from build123d import *

# Parameters (mm, degrees)
SKETCH1_W           = 85
SKETCH1_H           = 20
BOSS_EXTRUDE1_DEPTH = 3
SKETCH2_W           = 3
SKETCH2_H           = 20
BOSS_EXTRUDE2_DEPTH = 12
SKETCH3_W           = 49.5
SKETCH3_H           = 20
BOSS_EXTRUDE3_DEPTH = 3
SKETCH4_W           = 43.5
SKETCH4_H           = 3
CUT_EXTRUDE1_DEPTH  = 50.307707308
SKETCH5_R           = 3.1
CUT_EXTRUDE2_DEPTH  = 48.22552276
SKETCH6_R           = 1.6
CUT_EXTRUDE3_DEPTH  = 48.22552276
FILLET1_R           = 3


with BuildPart() as part:
    # Sketch1 → Boss-Extrude1 (new body)
    with BuildSketch(Plane.XY):
        Rectangle(SKETCH1_W, SKETCH1_H)
    extrude(amount=BOSS_EXTRUDE1_DEPTH)

    # Sketch2 → Boss-Extrude2 (add)
    with BuildSketch(Plane(origin=(0, 0, 0), x_dir=(-1, 0, 0), z_dir=(0, 0, -1))):
        with Locations((-23.25, 0)):
            Rectangle(SKETCH2_W, SKETCH2_H)
        with Locations((23.25, 0)):
            Rectangle(SKETCH2_W, SKETCH2_H)
    extrude(amount=BOSS_EXTRUDE2_DEPTH)

    # Sketch3 → Boss-Extrude3 (add)
    with BuildSketch(Plane(origin=(0, 0, -12), x_dir=(-1, 0, 0), z_dir=(0, 0, -1))):
        Rectangle(SKETCH3_W, SKETCH3_H)
    extrude(amount=BOSS_EXTRUDE3_DEPTH)

    # Sketch4 → Cut-Extrude1 (cut, through all)
    with BuildSketch(Plane.XZ.offset(10)):
        with Locations((0, 1.5)):
            Rectangle(SKETCH4_W, SKETCH4_H)
    extrude(amount=-CUT_EXTRUDE1_DEPTH, mode=Mode.SUBTRACT)

    # Sketch5 → Cut-Extrude2 (cut, through all)
    with BuildSketch(Plane(origin=(0, 0, -15), x_dir=(-1, 0, 0), z_dir=(0, 0, -1))):
        Circle(SKETCH5_R)
    extrude(amount=-CUT_EXTRUDE2_DEPTH, mode=Mode.SUBTRACT)

    # Sketch6 → Cut-Extrude3 (cut, through all)
    with BuildSketch(Plane.XY.offset(3)):
        with Locations((32.380648159, 0.030992543)):
            Circle(SKETCH6_R)
        with Locations((-32.619351841, 0.030992543)):
            Circle(SKETCH6_R)
    extrude(amount=-CUT_EXTRUDE3_DEPTH, mode=Mode.SUBTRACT)

    # Fillet1
    fillet1_edges = [part.edges().sort_by_distance(p)[0] for p in [
        (24.75, 0, -15),
        (-24.75, 0, -15),
        (42.5, -10, 1.5),
        (-42.5, -10, 1.5),
        (-42.5, 10, 1.5),
        (42.5, 10, 1.5),
    ]]
    fillet(fillet1_edges, radius=FILLET1_R)


solid = part.part
Model file for the job. Use its own axes, mm. A direction names the side the tool comes from. Give positions to 0.01 mm unless a question says otherwise; leave off trailing zeros. Loops run counter-clockwise (first coordinate to the right, second up) from the corner with the lowest first, then second, coordinate; pieces in that order, holes last.
1) Tool access for faces 4 (the cylindrical face through (41.6, -9.14, 1.52)), 5 (the flat face through (35, 0, 0)), 6 (the flat face through (21.75, 0, -5)), 7 (the flat face through (-24.75, 0, -6)), 8 (the flat face through (-42.5, 0, 1)): list every direction of +Z, -Z, +X, -X, +Y, -Y with a clear straight run to the whole face (end or side of a thin tool).
2) Saw through at D-D (x = -27). Write the cut outline in (y, z), plus the area to 3 significant figures.
3) Flat gauge pins, fed straight in: pin 1 Ø12 at (x, y) = (11.5, 3.5) entering from +Z; pin 2 Ø9.5 at (y, z) = (-5, -3.5) entering from +X; pin 3 Ø9 at (x, y) = (38, -4) entering from -Z; pin 4 Ø3.5 at (y, z) = (4, -3) entering from -X. Where does each tip first touch, or does it go through?
4) Pull direction X, two halves, no side cores. Call faces 1 (the cylindrical face through (-34.218, 0.101, 1.521)), 2 (the cylindrical face through (41.6, 9.14, 1.52)), 3 (the flat face through (0, -10, -13)): +X half, -X half, draft (parallel to the pull), parting line (faces both ways), or undercut.
5) Saw through at A-A (x = 0). Write the cut outline in (y, z).
6) Saw through at C-C (y = -5). Write the cut outline in (x, z), plus the area to 3 significant figures.
7) Saw through at B-B (z = -2.25). Write the cut outline in (x, y).
8) Wall check: line 1 (X direction, y = -1, z = -9); line 2 (X direction, y = -2, z = 2.5); line 3 (Y direction, x = 0, z = -13.1). Give the ranges that are in metal, low to high.
Answer block:
1. face 4: +Z, -Z, +X, -Y
1. face 5: -Z, +X, +Y, -Y
1. face 6: +Z, +Y, -Y
1. face 7: -Z, -X, +Y, -Y
1. face 8: +Z, -Z, -X, +Y, -Y
2. outline: (-10, 0) - (10, 0) - (10, 3) - (-10, 3) - close
2. area: 60.0 mm2
3. pin 1: stops at z = -12
3. pin 2: stops at x = 42.5
3. pin 3: stops at z = 0
3. pin 4: stops at x = -24.75
4. face 1: undercut
4. face 2: +X half
4. face 3: draft
5. outline: (-10, -15) - (-3.1, -15) - (-3.1, -12) - (-10, -12) - close; (3.1, -15) - (10, -15) - (10, -12) - (3.1, -12) - close
6. outline: (-42.5, 0) - (-24.75, 0) - (-24.75, -12) arc R3 ccw to (-21.75, -15) - (21.75, -15) arc R3 ccw to (24.75, -12) - (24.75, 0) - (42.5, 0) - (42.5, 3) - (21.75, 3) - (21.75, -12) - (-21.75, -12) - (-21.75, 3) - (-42.5, 3) - close
6. area: 341 mm2
7. outline: (-24.75, -10) - (-21.75, -10) - (-21.75, 10) - (-24.75, 10) - close; (21.75, -10) - (24.75, -10) - (24.75, 10) - (21.75, 10) - close
8. line 1: x = -24.75 to -21.75, 21.75 to 24.75
8. line 2: x = -42.5 to -21.75, 21.75 to 42.5
8. line 3: y = -10 to -3.1, 3.1 to 10
